The model under review builds one solid part; all positions refer to its coordinate system, in mm. A direction names the side the tool comes from. Coordinates: 2 decimals unless noted, no trailing zeros. Order: outer loops, then holes, each group sorted by start corner. A loop starts at its lowest first (then second) coordinate and runs counter-clockwise, first axis right, second up. Notation, with made-up numbers: (-19, -32) -> (35, -32) arc R22 cw to (35, -2) -> close; hole circle Ø6 at (-14, 26.5). An arc over 180 degrees is marked (long way). Use one line per item in the form item = value. Start each with the question number.
(1) Take a section at C-C (z = -2.5). State the section outline as (x, y) points, then the cut area to 3 significant figures.
(2) For faces 5 (the flat face through (-1, 2.429, 3)), 6 (the flat face through (3.979, -1, 3)), 7 (the flat face through (6, 6.644, 3)), list the 3-axis set-ups (+Z, -Z, +X, -X, +Y, -Y) from which the entire face can be reached by the end or side of a thin tool; tool diameter is ignored.
(3) Insertion check: pin 1 Ø1.6 at (y, z) = (7.5, 3.5) entering from -X; pin 2 Ø2 at (x, z) = (4.5, 1) entering from +Y; pin 3 Ø2.5 at (x, y) = (0, 6.858) entering from +Z; pin 4 Ø5.5 at (x, y) = (6, 3.5) entering from -Z. Each pin has a flat end and moves straight along its axis. Give the tip position at first contact, or say it passes through.
(4) Wall thickness on line 1 along Y through (x, z) = (0, 1.5); line 2 along Y through (x, z) = (7.25, 3.75); line 3 along Y through (x, z) = (1.25, -1): over which ranges is each line inside the solid? List them lowest first.
(5) Take a section at D-D (x = 3). State the section outline as (y, z) points.
(6) Mouldability with a two-part tool opening along Y and no side actions: class faces 1 (the flat face through (5, 9.144, 2)), 2 (the flat face through (8.979, 3.3, 1.5)), 3 (the cylindrical face through (4.62, 3.06, 0.99)), 4 (the cylindrical face through (0.032, 13.637, -2.285)) as +Y half, -Y half, draft (parallel to the pull), parting line (faces both ways), or undercut.
(7) Take a section at B-B (x = 0.5). State the section outline as (y, z) points.
(8) Take a section at A-A (y = 0). State the section outline as (x, z) points, then the cut area to 3 significant figures.
Autodesk Inventor part; units mm, degrees
ref_plane "YZ Plane" through (0, 0, 0) normal (1, 0, 0) x (0, 1, 0)
ref_plane "XZ Plane" through (0, 0, 0) normal (0, 1, 0) x (-1, 0, 0)
ref_plane "XY Plane" through (0, 0, 0) normal (0, 0, 1) x (1, 0, 0)
sketch "Sketch21" plane through (0, 0, 0) normal (0, 0, 1) x (1, 0, 0)
  line L0 (0, 0) -> (0, 6.858)
  line L1 (0, 6.858) -> (3.429, 6.858)
  line L2 (3.429, 6.858) -> (3.429, 3.434)
  line L3 (3.429, 3.434) -> (7.229, 3.434)
  circle A0 centre (0, 0) radius 1.651
  circle A1 centre (0, 6.858) radius 1.651
  circle A2 centre (3.429, 3.434) radius 1.25
  circle A3 centre (7.229, 3.434) radius 1.25
  line L4 (7.229, 3.434) -> (8.979, 3.434)
  line L5 (8.979, 9.144) -> (-2.286, 9.144)
  line L6 (-2.286, 9.144) -> (-2.286, -2.286)
  line L7 (-2.286, -2.286) -> (8.979, -2.286)
  line L8 (8.979, -2.286) -> (8.979, 9.144)
  dimension "d76" = 6.858
  dimension "d77" = 3.429
  dimension "d78" = 3.424
  dimension "d79" = 3.8
  dimension "d80" = 3.302
  dimension "d81" = 3.302
  dimension "d82" = 2.5
  dimension "d83" = 2.5
  dimension "d84" = 1.75
extrude "Extrusion19" add sketch "Sketch21" along normal blind 2
sketch "Sketch22" plane through (0, 0, 2) normal (0, 0, 1) x (1, 0, 0)
  line L0 (-2.286, -2.286) -> (8.979, -2.286)
  line L1 (8.979, -2.286) -> (3.979, -2.286)
  line L2 (3.979, -2.286) -> (3.979, 0.214)
  line L3 (3.979, 0.214) -> (8.979, 0.214)
  line L4 (8.979, 0.214) -> (8.979, -2.286)
  line L5 (8.979, 9.144) -> (-2.286, 9.144)
  line L6 (8.979, 9.144) -> (3.979, 9.144)
  line L7 (3.979, 9.144) -> (3.979, 6.644)
  line L8 (3.979, 6.644) -> (8.979, 6.644)
  line L9 (8.979, 6.644) -> (8.979, 9.144)
  line L10 (-2.286, 9.144) -> (-2.286, -2.286)
  line L11 (-2.286, 3.429) -> (-1.286, 3.429)
  line L12 (-1.286, 3.429) -> (-1.286, 4.429)
  line L13 (-1.286, 4.429) -> (-2.286, 4.429)
  line L14 (-2.286, 4.429) -> (-2.286, 3.429)
  line L15 (-2.286, 4.429) -> (-0.286, 4.429)
  line L16 (-0.286, 4.429) -> (-0.286, 2.429)
  line L17 (-0.286, 2.429) -> (-2.286, 2.429)
  line L18 (-2.286, 2.429) -> (-2.286, 4.429)
  point P0 (0, 0)
  dimension "d89" = 5
  dimension "d90" = 2.5
  dimension "d91" = 5
  dimension "d92" = 2.5
  dimension "d93" = 1
  dimension "d94" = 1
  dimension "d95" = 2
  dimension "d96" = 2
extrude "Extrusion20" add sketch "Sketch22" along normal blind 2
sketch "Sketch23" plane through (0, 0, 0) normal (0, 0, -1) x (-1, 0, 0)
  circle A0 centre (0, 6.858) radius 1.651
  circle A1 centre (0, 6.858) radius 2.286
  line L0 (2.286, 9.144) -> (2.286, -2.286)
  line L1 (-2.286, 6.858) -> (-2.286, -2.286)
  line L2 (-8.979, 9.144) -> (2.286, 9.144)
  line L3 (-2.286, -2.286) -> (2.286, -2.286)
  line L4 (2.286, -2.286) -> (2.286, 9.144)
  line L5 (2.286, 9.144) -> (-2.286, 9.144)
  line L6 (-2.286, 9.144) -> (-2.286, -2.286)
  circle A2 centre (0, 0) radius 1.651
extrude "Extrusion21" add sketch "Sketch23" along normal blind 5
sketch "Sketch24" plane through (2.286, 2.928, 0) normal (1, 0, 0) x (0, 0, -1)
  line L0 (5, -5.214) -> (5, 6.216)
  line L1 (5, 6.216) -> (-2, 6.216)
  line L2 (5, -5.214) -> (5, 6.216)
  line L3 (5, 0.501) -> (-9.7149, 0.501)
  line L4 (0, 1.012) -> (0, 0)
  line L5 (0, 0.506) -> (5, 0.501)
  circle A0 centre (2.5, 0.5035) radius 1.651
  point P0 (0, -2.928)
  dimension "d101" = 3.302
extrude "Extrusion22" cut sketch "Sketch24" against normal blind 5 contours A0 L3 | L3 A0
sketch "Sketch25" plane through (2.286, 2.928, 0) normal (1, 0, 0) x (0, 0, -1)
  circle A0 centre (2.5, 0.5035) radius 1.651
  line L0 (5, 6.216) -> (-2, 6.216)
  line L1 (5, -5.214) -> (5, 6.216)
  circle A1 centre (2.5, 9.0723) radius 1.651
  line L2 (5, 11.9285) -> (0, 11.9285)
  line L3 (0, 11.9285) -> (0, 6.216)
  line L4 (0, 6.216) -> (5, 6.216)
  line L5 (5, 6.216) -> (5, 11.9285)
  point P0 (0, -2.928)
  dimension "d105" = 3.302
extrude "Extrusion23" add sketch "Sketch25" against normal blind 5 contours L0 L3 L2 L5
sketch "Sketch26" plane through (-2.714, 9.144, 0) normal (0, -1, 0) x (1, 0, 0)
  line L0 (0.428, 0) -> (0, 0)
  line L1 (5, -5) -> (0.428, -5)
  line L2 (0, 0) -> (0.428, 0)
  line L3 (0.428, 0) -> (0.428, -5)
  line L4 (0.428, -5) -> (0, -5)
  line L5 (0, -5) -> (0, 0)
  point P0 (2.714, 0)
extrude "Extrusion24" cut sketch "Sketch26" against normal blind 50
properties part number "SensorMount"
Findings:
q1.outline = (-2.29, -2.29) -> (2.29, -2.29) -> (2.29, 1.78) -> (-2.29, 1.78) -> close; (-2.29, 5.08) -> (2.29, 5.08) -> (2.29, 10.35) -> (-2.29, 10.35) -> close; (-2.29, 13.65) -> (2.29, 13.65) -> (2.29, 14.86) -> (-2.29, 14.86) -> close; hole circle Ø3.3 at (0, 0); hole circle Ø3.3 at (0, 6.86)
q1.area = 31.1 mm²
q2.face_5 = +Z, +X, -X, -Y
q2.face_6 = +Z, -X, +Y, -Y
q2.face_7 = +Z, +X, -X
q3.pin_1 = 3.98
q3.pin_2 = 9.14
q3.pin_3 = through
q3.pin_4 = 0
q4.line_1 = -2.29 to -1.65, 1.65 to 5.21, 8.51 to 9.14
q4.line_2 = -2.29 to 0.21, 6.64 to 9.14
q4.line_3 = -2.29 to -1.08, 1.08 to 2.74, 4.12 to 5.78, 7.94 to 11.31, 12.69 to 14.86
q5.outline = (-2.29, 0) -> (2.26, 0) -> (2.26, 2) -> (-2.29, 2) -> close; (4.61, 0) -> (9.14, 0) -> (9.14, 2) -> (4.61, 2) -> close
q6.face_1 = +Y half
q6.face_2 = draft
q6.face_3 = undercut
q6.face_4 = undercut
q7.outline = (-2.29, -5) -> (-1.57, -5) -> (-1.57, 2) -> (-2.29, 2) -> close; (1.57, -5) -> (5.28, -5) -> (5.28, 2) -> (1.57, 2) -> close; (8.43, -5) -> (14.86, -5) -> (14.86, 0) -> (9.14, 0) -> (9.14, 2) -> (8.43, 2) -> close; hole circle Ø3.3 at (3.43, -2.5); hole circle Ø3.3 at (12, -2.5)
q8.outline = (-2.29, -5) -> (-1.65, -5) -> (-1.65, 2) -> (-2.29, 2) -> close; (1.65, -5) -> (2.29, -5) -> (2.29, 0) -> (8.98, 0) -> (8.98, 4) -> (3.98, 4) -> (3.98, 2) -> (1.65, 2) -> close
q8.area = 32.3 mm²
